CAD build for the part. Positions are in the model's coordinates, mm. A direction names the side the tool comes from. Round coordinates to 2 decimals unless told otherwise and drop trailing zeros. Order: outer loops, then holes, each group sorted by start corner. A loop starts at its lowest first (then second) coordinate and runs counter-clockwise, first axis right, second up. Notation, with made-up numbers: M -39.5,65.25 L 15.5,65.25 A16 cw 15.5,87.25 Z; hole C -15.75,82.25 d6. An arc over 180 degrees is marked long. Answer as a JSON object with one key per item and string values.
```python
from build123d import *

# Parameters (mm, degrees)
SKETCH1_R           = 20
BOSS_EXTRUDE1_DEPTH = 3
BOSS_EXTRUDE2_DEPTH = 30
FILLET1_R           = 2
SKETCH3_R           = 21
BOSS_EXTRUDE3_DEPTH = 7
BOSS_EXTRUDE4_START = -3
SKETCH4_R           = 20
BOSS_EXTRUDE4_DEPTH = 3
SKETCH5_R           = 8.5
CUT_EXTRUDE1_DEPTH  = 43
SKETCH6_R           = 16
CUT_EXTRUDE2_DEPTH  = 43


with BuildPart() as part:
    # Sketch1 → Boss-Extrude1 (new body)
    with BuildSketch(Plane.XY):
        Circle(SKETCH1_R)
    extrude(amount=-BOSS_EXTRUDE1_DEPTH)

    # Sketch2 → Boss-Extrude2 (add)
    with BuildSketch(Plane.XY):
        with BuildLine():
            Line((22.995189637, 3.5), (35.372983102, 3.5))
            Line((35.372983102, 3.5), (35.372983102, -3.5))
            Line((35.372983102, -3.5), (22.995189637, -3.5))
            add(Edge.make_bspline(
                [(-10.012259603, -15.596019766), (-7.820118135, -12.904569359), (3.188583593, -8.31405085), (13.833155486, -3.052585892), (22.995189637, -3.5)],
                knots=[0, 0, 0, 0, 0.276488418, 1, 1, 1, 1], degree=3))
            ThreePointArc((-10.012259603, -15.596019766), (-18.533245126, 0), (-10.012259603, 15.596019766))
            add(Edge.make_bspline(
                [(-10.012259603, 15.596019766), (-7.820118135, 12.904569359), (3.188583593, 8.31405085), (13.833155486, 3.052585892), (22.995189637, 3.5)],
                knots=[0, 0, 0, 0, 0.276488418, 1, 1, 1, 1], degree=3))
        make_face()
    extrude(amount=-BOSS_EXTRUDE2_DEPTH)

    # Fillet1
    fillet1_edges = [part.edges().sort_by_distance(p)[0] for p in [
        (-10.012259603, 15.596019766, -16.5),
        (-10.012259603, -15.596019766, -16.5),
    ]]
    fillet(fillet1_edges, radius=FILLET1_R)

    # Sketch3 → Boss-Extrude3 (add)
    with BuildSketch(Plane.XZ.offset(3.5)):
        with Locations((47.699784797, -15.04571332)):
            Circle(SKETCH3_R)
    extrude(amount=-BOSS_EXTRUDE3_DEPTH)

    # Sketch4 → Boss-Extrude4 (add)
    with BuildSketch(Plane(origin=(0, 0, -30), x_dir=(-1, 0, 0), z_dir=(0, 0, -1)).offset(BOSS_EXTRUDE4_START)):
        Circle(SKETCH4_R)
    extrude(amount=BOSS_EXTRUDE4_DEPTH)

    # Sketch5 → Cut-Extrude1 (cut)
    with BuildSketch(Plane.XY):
        Circle(SKETCH5_R)
    extrude(amount=-CUT_EXTRUDE1_DEPTH, mode=Mode.SUBTRACT)

    # Sketch6 → Cut-Extrude2 (cut)
    with BuildSketch(Plane.XZ.offset(3.5)):
        with Locations((47.699784797, -15.04571332)):
            Circle(SKETCH6_R)
    extrude(amount=-CUT_EXTRUDE2_DEPTH, mode=Mode.SUBTRACT)


solid = part.part
```
Item 1: Wall check: line 1 along Z through (x, y) = (2, 10.5); line 2 along X through (y, z) = (2.5, -3.5); line 3 along Y through (x, z) = (-3.5, -19). Give the ranges that are in metal, low to high. Write a range as [from, to].
Worked answers:
{"line 1": "z = [-30, -27], [-3, 0]", "line 2": "x = [-18.36, -8.12], [8.12, 36.62], [58.78, 65.24]", "line 3": "y = [-11.08, -7.75], [7.75, 11.08]"}
Item 2: Saw through at A-A on y = 0. List the corners of the cut face in (x, z).
Worked answers:
{"outline": "M -20,-30 L -8.5,-30 L -8.5,0 L -20,0 L -20,-3 L -18.53,-3 L -18.53,-27 L -20,-27 Z; M 8.5,-30 L 32.96,-30 A21 ccw long 33.05,0 L 8.5,0 Z; hole C 47.7,-15.05 d32"}
Item 3: Drop flat-ended pins along their axis: pin 1 Ø12 at (x, z) = (1.5, -30.5) entering from -Y; pin 2 Ø15.5 at (x, y) = (0, 0) entering from +Z; pin 3 Ø5 at (y, z) = (3, -23.5) entering from -X; pin 4 Ø10 at (x, z) = (7.5, -14.5) entering from -Y. Give the stop position or say it passes through.
Worked answers:
{"pin 1": "stops at y = -20", "pin 2": "passes through", "pin 3": "stops at x = -18.53", "pin 4": "stops at y = -8.44"}
Item 4: Two-plate mould, pull along Z, no slides. Class faces 6 (the cylindrical face through (-18.53, -0.23, -14.83)), 7 (the cylindrical face through (-19.983, 0.83, -1.479)), 8 (the flat face through (1, 9, -30)): released by +Z, released by -Z, zero draft, split by the parting line, or undercut.
Worked answers:
{"face 6": "undercut", "face 7": "zero draft", "face 8": "released by -Z"}
Item 5: Saw through at D-D on x = 62. List the corners of the cut face in (y, z).
Worked answers:
{"outline": "M -3.5,-30.42 L 3.5,-30.42 L 3.5,-22.22 L -3.5,-22.22 Z; M -3.5,-7.87 L 3.5,-7.87 L 3.5,0.33 L -3.5,0.33 Z"}
Item 6: Saw through at C-C on z = -25.5. State how many separate pieces and enclosed holes the cut face has, and give its area (3 significant figures).
Worked answers:
{"separate pieces": "2", "enclosed holes": "1", "area": "585 mm2"}
Item 7: 3-axis set-ups, long thin cutter, end or side, ignore diameter. For faces 1 (the flat face through (30, -3.5, -15)), 2 (the cylindrical face through (-19.983, -0.83, -28.479)), 3 (the flat face through (30, 3.5, -15)), 4 (the cylindrical face through (55.08, -0.05, -29.24)), 5 (the flat face through (1, -9, 0)): which of +Z, -Z, +X, -X, +Y, -Y reach the whole face in a straight line?
Worked answers:
{"face 1": "+Z, -Z, +X, -Y", "face 2": "+Z, -Z", "face 3": "+Z, -Z, +X, +Y", "face 4": "+Y, -Y", "face 5": "+Z, -X, +Y, -Y"}
Item 8: Saw through at B-B on x = 52.5. List the corners of the cut face in (y, z), and give its area (3 significant figures).
Worked answers:
{"outline": "M -3.5,-35.49 L 3.5,-35.49 L 3.5,-30.31 L -3.5,-30.31 Z; M -3.5,0.22 L 3.5,0.22 L 3.5,5.4 L -3.5,5.4 Z", "area": "72.5 mm2"}
